Autodesk Inventor part; units mm, degrees
ref_plane "Work Plane1" through (-0.0642, 19.0883, -82.55) normal (-1, 0, 0) x (0, 0, 1)
ref_plane "YZ Plane" through (0, 0, 0) normal (1, 0, 0) x (0, 1, 0)
ref_plane "XZ Plane" through (0, 0, 0) normal (0, 1, 0) x (-1, 0, 0)
sketch "Sketch1" plane through (0, 0, 0) normal (0, 1, 0) x (-1, 0, 0)
  line L0 (-76.2, 57.15) -> (76.2, 57.15)
  line L1 (76.2, 57.15) -> (76.2, -57.15)
  line L2 (76.2, -57.15) -> (-76.2, -57.15)
  line L3 (-76.2, -57.15) -> (-76.2, 57.15)
  line L4 (-76.2, 57.15) -> (76.2, -57.15) construction
  line L5 (76.2, 57.15) -> (-76.2, -57.15) construction
  point P0 (0, 0)
  dimension "d0" = 152.4
  dimension "d1" = 114.3
extrude "Extrusion1" add sketch "Sketch1" along normal blind 9.55
sketch "Sketch2" plane through (0, 9.55, 0) normal (0, 1, 0) x (1, 0, 0)
  line L0 (54, -57.15) -> (-54, -57.15)
  line L1 (-54, -57.15) -> (-54, 57.15)
  line L2 (-54, 57.15) -> (54, 57.15)
  line L3 (54, 57.15) -> (54, -57.15)
  line L4 (54, -57.15) -> (-54, 57.15) construction
  line L5 (-54, -57.15) -> (54, 57.15) construction
  point P0 (0, 0)
  dimension "d4" = 108
  dimension "d5" = 114.3
extrude "Extrusion2" add sketch "Sketch2" along normal blind 9.55
fillet "Fillet1" radius 8 1 edges at (-54, 9.55, 0)
fillet "Fillet2" radius 8 1 edges at (54, 9.55, 0)
sketch "Sketch3" plane through (-76.2, 0, 57.15) normal (0, 0, 1) x (1, 0, 0)
  line L0 (0, 0) -> (0, 9.55) construction
  line L1 (0, 9.55) -> (0, 14.325) construction
  line L2 (0, 14.325) -> (152.4, 14.325) construction
  circle A0 centre (39.2, 14.325) radius 4.7625
  circle A1 centre (64.2, 14.325) radius 4.7625
  circle A2 centre (88.2, 14.325) radius 4.7625
  circle A3 centre (113.2, 14.325) radius 4.7625
  arc A4 (130.2, 17.55) -> (138.2, 9.55) centre (138.2, 17.55) ccw
  arc A5 (14.2, 9.55) -> (22.2, 17.55) centre (14.2, 17.55) ccw
  point P0 (76.2, 0)
  dimension "d10" = 9.55
  dimension "d11" = 4.775
  dimension "d12" = 152.4
  dimension "d13" = 9.525
  dimension "d14" = 9.525
  dimension "d15" = 9.525
  dimension "d16" = 9.525
  dimension "d17" = 25
  dimension "d18" = 25
  dimension "d19" = 25
  dimension "d20" = 25
extrude "Extrusion3" add sketch "Sketch3" along normal blind 20
sketch "Sketch4" plane through (-37, 14.325, 77.15) normal (0, 0, 1) x (1, 0, 0)
  line L0 (-0.0011, 4.7559) -> (25.2383, 4.7559)
  line L1 (25.2383, 4.7559) -> (25.2383, -4.6618)
  line L2 (25.2383, -4.6618) -> (-0.0011, -4.6618)
  line L3 (-0.0011, -4.6618) -> (-0.0011, 4.7559)
  point P0 (37, -14.325)
extrude "Extrusion4" add sketch "Sketch4" along normal blind 5.4
sketch "Sketch5" plane through (12, 14.325, 77.15) normal (0, 0, 1) x (1, 0, 0)
  line L0 (0.0017, 4.7559) -> (25.0231, 4.7559)
  line L1 (25.0231, 4.7559) -> (25.0231, -4.7498)
  line L2 (25.0231, -4.7498) -> (0.0017, -4.7498)
  line L3 (0.0017, -4.7498) -> (0.0017, 4.7559)
  point P0 (-12, -14.325)
extrude "Extrusion5" add sketch "Sketch5" along normal blind 5.4
sketch "Sketch6" plane through (76.2, 0, -57.15) normal (0, 0, -1) x (-1, 0, 0)
  circle A0 centre (39.2, 14.325) radius 4.7625
  circle A1 centre (113.2, 14.325) radius 4.7625
  circle A2 centre (39.2, 14.325) radius 4.7625
  circle A3 centre (113.2, 14.325) radius 4.7625
  point P0 (76.2, 0)
extrude "Extrusion6" add sketch "Sketch6" along normal blind 76.2
sketch "Sketch7" plane through (76.2, 0, -57.15) normal (0, 0, -1) x (-1, 0, 0)
  circle A0 centre (64.2, 14.325) radius 4.7625
  circle A1 centre (88.2, 14.325) radius 4.7625
  circle A2 centre (64.2, 14.325) radius 4.7625
  circle A3 centre (88.2, 14.325) radius 4.7625
  point P0 (76.2, 0)
extrude "Extrusion7" add sketch "Sketch7" along normal blind 20
sketch "Sketch8" plane through (12, 14.325, -77.15) normal (0, 0, -1) x (-1, 0, 0)
  line L0 (-0.0002, 4.7633) -> (24.1286, 4.7633)
  line L1 (24.1286, 4.7633) -> (24.1286, -4.7128)
  line L2 (24.1286, -4.7128) -> (-0.0002, -4.7128)
  line L3 (-0.0002, -4.7128) -> (-0.0002, 4.7633)
  point P0 (12, -14.325)
extrude "Extrusion8" add sketch "Sketch8" along normal blind 5.4
sketch "Sketch9" plane through (0, 9.55, 0) normal (0, 1, 0) x (1, 0, 0)
  line L0 (-76.2, 57.15) -> (-76.2, -57.15) construction
  line L1 (-76.2, -57.15) -> (-62, -57.15) construction
  line L2 (-62, 57.15) -> (-62, -57.15) construction
  line L3 (-62, 57.15) -> (-76.2, 57.15) construction
  line L4 (76.2, 57.15) -> (62, 57.15) construction
  line L5 (76.2, -57.15) -> (76.2, 57.15) construction
  line L6 (62, -57.15) -> (62, 57.15) construction
  line L7 (62, -57.15) -> (76.2, -57.15) construction
  line L8 (-76.2, -57.15) -> (-62, -57.15) construction
  line L9 (-69.1, 0) -> (-69.1, -25.4) construction
  line L10 (-69.1, 0) -> (-69.1, 25.4) construction
  circle A0 centre (-69.1, 25.4) radius 3.365
  circle A1 centre (-69.1, -25.4) radius 3.365
  point P0 (0, 0)
  dimension "d36" = 25.4
  dimension "d37" = 25.4
  dimension "d38" = 6.73
  dimension "d39" = 6.73
extrude "Extrusion9" cut sketch "Sketch9" against normal blind 10
ref_plane "Work Plane1" through (-0.0642, 19.0883, -82.55) normal (-1, 0, 0) x (0, 0, 1)
mirror "Mirror1" about plane through (-0.0642, 19.0883, -82.55) normal (-1, 0, 0) of "Extrusion9"
properties part number "cooling plate"
Source: CAD feature listing. Evaluate the final solid. Frame: model axes, mm. A direction names the side the tool comes from. Give positions to 0.01 mm unless a question says otherwise; leave off trailing zeros. Order: outer loops, then holes, each group sorted by start corner. A loop starts at its lowest first (then second) coordinate and runs counter-clockwise, first axis right, second up.
(1) Pull-direction query (X, two-part tool) for faces 1 (the face through (-56.281, 11.956, -0.8)), 2 (the face through (0, 14, -82.55)), 3 (the face through (37, 14, -133.35)); classes: +X half, -X half, draft (parallel to the pull), parting line (faces both ways), or undercut.
(2) Section query A-A (x = 21). Return the cut outline in (y, z).
(3) Contact query for flat-ended pins moving along their axis: P1, Ø11, axis at x = 68.97, z = -25.4, coming from the -Y side; P2, Ø6, axis at x = -5.5, z = -80.5, coming from the +Y side; P3, Ø10, axis at y = 14.5, z = -77, coming from the +X side; P4, Ø6, axis at x = 2.5, y = 15.5, coming from the -Z side. Output: stop coordinate, or through.
(4) Section query B-B (x = -69.1). Return the cut outline in (y, z) (3 decimals).
(5) Section query D-D (x = -28). Return the cut outline in (y, z), plus the area to 3 significant figures.
(6) Access query for faces 4 (the face through (69, 9.55, 1)), 5 (the face through (37.023, 14, 80)), 6 (the face through (33.22, 17.22, 67.01)). Directions: +Z, -Z, +X, -X, +Y, -Y. A direction counts if a zero-diameter tool reaches every point of the face in a straight line with its end or side. Return the directions, or none.
(7) Material intervals for line 1 along X through (y, z) = (4.5, -25.4) (3 decimals); line 2 along Z through (x, y) = (-69.1, 7.5) (3 decimals); line 3 along Z through (x, y) = (-16, 6), sorted ascending.
(8) Section query C-C (z = -25.4). Return the cut outline in (x, y) (3 decimals), plus the area to 3 significant figures.
Outcome:
1. face 1: -X half
1. face 2: undercut
1. face 3: draft
2. outline: (0, -57.15) - (19.1, -57.15) - (19.1, 57.15) - (0, 57.15) - close; (9.58, 77.15) - (19.08, 77.15) - (19.08, 82.55) - (9.58, 82.55) - close
3. P1: stops at y = 0
3. P2: stops at y = 19.09
3. P3: stops at x = 41.76
3. P4: stops at z = -82.55
4. outline: (0, -57.15) - (9.55, -57.15) - (9.55, -28.765) - (0, -28.765) - close; (0, -22.035) - (9.55, -22.035) - (9.55, 22.035) - (0, 22.035) - close; (0, 28.765) - (9.55, 28.765) - (9.55, 57.15) - (0, 57.15) - close
5. outline: (0, -57.15) - (19.1, -57.15) - (19.1, 57.15) - (0, 57.15) - close; (9.66, 77.15) - (19.08, 77.15) - (19.08, 82.55) - (9.66, 82.55) - close
5. area: 2,230 mm2
6. face 4: +Z, -Z, +X, +Y
6. face 5: +Z, +X, +Y, -Y
6. face 6: none
7. line 1: x = -76.2 to -72.465, -65.735 to 65.607, 72.337 to 76.2
7. line 2: z = -57.15 to -28.765, -22.035 to 22.035, 28.765 to 57.15
7. line 3: z = -57.15 to 57.15
8. outline: (-76.2, 0) - (-72.465, 0) - (-72.465, 9.55) - (-76.2, 9.55) - close; (-65.735, 0) - (65.607, 0) - (65.607, 9.55) - (62, 9.55) arc R8 cw to (54, 17.55) - (54, 19.1) - (-54, 19.1) - (-54, 17.55) arc R8 cw to (-62, 9.55) - (-65.735, 9.55) - close; (72.337, 0) - (76.2, 0) - (76.2, 9.55) - (72.337, 9.55) - close
8. area: 2,390 mm2
